Could you check a few things on this model? Use its own coordinates, in mm. Coordinates: 2 decimals unless noted, no trailing zeros. Write each loop counter-clockwise with the first axis right and the second up, starting at its lowest first coordinate (ties: lowest second). Pieces come first, ordered by that corner, then holes.
Item 1: I want a section at B-B on x = 15. Please give me the cut outline in (y, z), then the cut area to 3 significant figures.
Item 2: I want a section at C-C on z = 2.5. State how many separate pieces and enclosed holes the cut face has, then the cut area to 3 significant figures.
Item 3: I want a section at D-D on y = -38.1. Please give me the cut outline in (x, z), then the cut area to 3 significant figures.
Item 4: Thinking about a two-plate mould opening in X: for faces 1 (the flat face through (-1, 1, 0)), 2 (the cylindrical face through (56.804, 36.269, 3.219)), 3 (the cylindrical face through (-18.3, 0.1, 3.2)), 4 (the flat face through (-76.2, -1, 3)), which applies, +X half, -X half, draft (parallel to the pull), parting line (faces both ways), or undercut?
Item 5: If I drill on probe 1 along X at (y, z) = (38, 1.5); probe 2 along X at (y, z) = (41, 0.5); probe 3 along Y at (x, z) = (15, 3.5), over which ranges is the centre line in solid material (lowest first)?
Item 6: I want a section at A-A on y = 0. Please give me the cut outline in (x, z).
from build123d import *

# Parameters (mm, degrees)
F0_W     = 152.4
F0_H     = 101.6
F1_DEPTH = 6.35
F2_R     = 4.78155
F3_DEPTH = 6.35
F5_DEPTH = 6.351
F6_R     = 3.3
F7_DEPTH = 6.351


with BuildPart() as f1:
    # F0 (on Top) → F1 (new body)
    with BuildSketch(Plane.XY):
        Rectangle(F0_W, F0_H)
    extrude(amount=F1_DEPTH)

    # F2 (on face) → F3 (cut, through all)
    with BuildSketch(Plane.XY.offset(6.35)):
        with Locations((-52.3875, 38.1)):
            Circle(F2_R)
        with Locations((52.3875, 38.1)):
            Circle(F2_R)
        with Locations((-52.3875, -38.1)):
            Circle(F2_R)
        with Locations((52.3875, -38.1)):
            Circle(F2_R)
    extrude(amount=-F3_DEPTH, mode=Mode.SUBTRACT)

    # F4 (on face) → F5 (cut, through all)
    with BuildSketch(Plane.XY.offset(6.35)):
        with BuildLine():
            Line((-34.217194, -3.570841), (-34.13125, -3.571875))
            ThreePointArc((-34.13125, -3.571875), (-34.088275, 3.571616), (-34.217194, -3.570841))
        make_face()
        with BuildLine():
            Line((34.13125, -3.571875), (34.275124, -3.568976))
            ThreePointArc((34.275124, -3.568976), (34.059298, 3.57115), (34.13125, -3.571875))
        make_face()
    extrude(amount=-F5_DEPTH, mode=Mode.SUBTRACT)

    # F6 (on face) → F7 (cut, through all)
    with BuildSketch(Plane.XY.offset(6.35)):
        with Locations((-15, 0)):
            Circle(F6_R)
        with Locations((15, 0)):
            Circle(F6_R)
    extrude(amount=-F7_DEPTH, mode=Mode.SUBTRACT)


solid = f1.part
Response values:
1. outline: (-50.8, 0) - (-3.3, 0) - (-3.3, 6.35) - (-50.8, 6.35) - close; (3.3, 0) - (50.8, 0) - (50.8, 6.35) - (3.3, 6.35) - close
1. area: 603 mm2
2. separate pieces: 1
2. enclosed holes: 8
2. area: 15,000 mm2
3. outline: (-76.2, 0) - (-57.17, 0) - (-57.17, 6.35) - (-76.2, 6.35) - close; (-47.61, 0) - (47.61, 0) - (47.61, 6.35) - (-47.61, 6.35) - close; (57.17, 0) - (76.2, 0) - (76.2, 6.35) - (57.17, 6.35) - close
3. area: 846 mm2
4. face 1: draft
4. face 2: undercut
4. face 3: undercut
4. face 4: -X half
5. probe 1: x = -76.2 to -57.17, -47.61 to 47.61, 57.17 to 76.2
5. probe 2: x = -76.2 to -56.19, -48.59 to 48.59, 56.19 to 76.2
5. probe 3: y = -50.8 to -3.3, 3.3 to 50.8
6. outline: (-76.2, 0) - (-37.7, 0) - (-37.7, 6.35) - (-76.2, 6.35) - close; (-30.56, 0) - (-18.3, 0) - (-18.3, 6.35) - (-30.56, 6.35) - close; (-11.7, 0) - (11.7, 0) - (11.7, 6.35) - (-11.7, 6.35) - close; (18.3, 0) - (30.56, 0) - (30.56, 6.35) - (18.3, 6.35) - close; (37.7, 0) - (76.2, 0) - (76.2, 6.35) - (37.7, 6.35) - close
